Can you work these out from the model? Positions are in its coordinate system, mm. Give positions to 0.01 mm unless a question says otherwise; leave off trailing zeros. Loops run counter-clockwise (first coordinate to the right, second up) from the corner with the lowest first, then second, coordinate; pieces in that order, holes last. Notation, with made-up numbers: (-1, -2.5) - (54, -2.5) arc R18 cw to (54, 15.5) - close; hole circle Ø9 at (24, 44). An arc over 180 degrees is marked (long way). Write item = value, one per line.
from build123d import *

# Parameters (mm, degrees)
EXTRUSION3_DEPTH = 0.3
ESQUISSE2_W      = 12
ESQUISSE2_H      = 15
EXTRUSION4_DEPTH = 0.2


with BuildPart() as part:
    # Esquisse1 → Extrusion3 (new body)
    with BuildSketch(Plane.XY):
        with BuildLine():
            Line((-12.832841813, 25.021420219), (-12.832841813, 25.437540043))
            ThreePointArc((-12.832841813, 25.437540043), (-13.819409399, 26.424107629), (-14.805976985, 25.437540043))
            Line((-14.805976985, 25.437540043), (-14.805976985, 25.037540043))
            ThreePointArc((-14.805976985, 25.037540043), (-15.667751578, 24.60975507), (-16.333846188, 23.915512028))
            ThreePointArc((-16.333846188, 23.915512028), (-16.688617291, 23.169755053), (-16.810405862, 22.352942012))
            Line((-16.810405862, 22.352942012), (-16.810405862, 20.131551422))
            Line((-16.810405862, 20.131551422), (-17.410405862, 20.131551422))
            Line((-17.410405862, 20.131551422), (-17.410405862, 19.131551422))
            Line((-17.410405862, 19.131551422), (-14.810405862, 19.131551422))
            ThreePointArc((-14.810405862, 19.131551422), (-13.810405862, 18.131551422), (-12.810405862, 19.131551422))
            Line((-12.810405862, 19.131551422), (-10.210405862, 19.131551422))
            Line((-10.210405862, 19.131551422), (-10.210405862, 20.131551422))
            Line((-10.210405862, 20.131551422), (-10.810405862, 20.131551422))
            Line((-10.810405862, 20.131551422), (-10.810405862, 22.331551422))
            ThreePointArc((-10.810405862, 22.331551422), (-11.372418001, 24.014230931), (-12.832841813, 25.021420219))
        make_face()
        with BuildLine():
            Line((-11.310405862, 22.331551422), (-11.310405862, 19.631551422))
            Line((-11.310405862, 19.631551422), (-13.310405862, 19.631551422))
            Line((-13.310405862, 19.631551422), (-13.310405862, 19.131551422))
            ThreePointArc((-13.310405862, 19.131551422), (-13.810405862, 18.631551422), (-14.310405862, 19.131551422))
            Line((-14.310405862, 19.131551422), (-14.310405862, 19.631551422))
            Line((-14.310405862, 19.631551422), (-16.310405862, 19.631551422))
            Line((-16.310405862, 19.631551422), (-16.310405862, 22.352942012))
            ThreePointArc((-16.310405862, 22.352942012), (-16.21036525, 23.023895582), (-15.91894613, 23.636481668))
            ThreePointArc((-15.91894613, 23.636481668), (-15.220043493, 24.309156929), (-14.305976985, 24.633871146))
            Line((-14.305976985, 24.633871146), (-14.305976985, 25.437540043))
            ThreePointArc((-14.305976985, 25.437540043), (-13.819409399, 25.924107629), (-13.332841813, 25.437540043))
            Line((-13.332841813, 25.437540043), (-13.332841813, 24.614741777))
            ThreePointArc((-13.332841813, 24.614741777), (-11.888721032, 23.856609238), (-11.310405862, 22.331551422))
        make_face(mode=Mode.SUBTRACT)
    extrude(amount=EXTRUSION3_DEPTH)

    # Esquisse2 → Extrusion4 (add)
    with BuildSketch(Plane(origin=(0, 0, 0), x_dir=(-1, 0, 0), z_dir=(0, 0, -1))):
        with Locations((13.810405862, 22.167730135)):
            Rectangle(ESQUISSE2_W, ESQUISSE2_H)
    extrude(amount=EXTRUSION4_DEPTH)


solid = part.part
Q1. Imagine slicing it at A-A, the plane z = 0.15. Write out the boundary of the cut face in (x, y), then the cut area to 3 significant figures.
Output:
outline = (-17.41, 19.13) - (-14.81, 19.13) arc R1 ccw to (-12.81, 19.13) - (-10.21, 19.13) - (-10.21, 20.13) - (-10.81, 20.13) - (-10.81, 22.33) arc R2.8 ccw to (-12.83, 25.02) - (-12.83, 25.44) arc R0.99 ccw to (-14.81, 25.44) - (-14.81, 25.04) arc R2.8 ccw to (-16.81, 22.35) - (-16.81, 20.13) - (-17.41, 20.13) - close; hole (-16.31, 19.63) - (-14.31, 19.63) - (-14.31, 19.13) arc R0.5 ccw to (-13.31, 19.13) - (-13.31, 19.63) - (-11.31, 19.63) - (-11.31, 22.33) arc R2.3 ccw to (-13.33, 24.61) - (-13.33, 25.44) arc R0.49 ccw to (-14.31, 25.44) - (-14.31, 24.63) arc R2.3 ccw to (-16.31, 22.35) - close
area = 12.8 mm2
Q2. Imagine slicing it at D-D, the plane x = -13.75. Write out the boundary of the cut face in (y, z), then the cut area to 3 significant figures.
Output:
outline = (14.67, -0.2) - (29.67, -0.2) - (29.67, 0) - (26.42, 0) - (26.42, 0.3) - (25.92, 0.3) - (25.92, 0) - (18.64, 0) - (18.64, 0.3) - (18.13, 0.3) - (18.13, 0) - (14.67, 0) - close
area = 3.30 mm2
Q3. Imagine slicing it at B-B, the plane x = -17. Write out the boundary of the cut face in (y, z), then the cut area to 3 significant figures.
Output:
outline = (14.67, -0.2) - (29.67, -0.2) - (29.67, 0) - (20.13, 0) - (20.13, 0.3) - (19.13, 0.3) - (19.13, 0) - (14.67, 0) - close
area = 3.30 mm2
Q4. I need wall thicknesses on L1, parallel to X at y = 20, z = 0.1; L2, parallel to X at y = 21.75, z = 0.25; L3, parallel to Z at x = -16, y = 18.75. Which ranges of each line are inside material? Lowest first, please.
Output:
L1 = -17.41 to -16.31, -11.31 to -10.21
L2 = -16.81 to -16.31, -11.31 to -10.81
L3 = -0.2 to 0
Q5. We'd pull the mould along Y, two halves only. Please class faces 1 (the flat face through (-14, 22, 0)), 2 (the flat face through (-14, 22, -0.2)): released by +Y, released by -Y, zero draft, split by the parting line, or undercut.
Output:
face_1 = undercut
face_2 = zero draft
Q6. For pin 1 (1.5 mm diameter, centred on x = -13, y = 21.5, fed in from +Z); pin 2 (5 mm diameter, centred on x = -18, y = 19.5, fed in from +Z), each with a flat end and sliding along its axis, tell me the tip position at first contact or that it passes through.
Output:
pin_1 = 0
pin_2 = 0.3
Q7. Imagine slicing it at C-C, the plane y = 28.75. Write out the boundary of the cut face in (x, z).
Output:
outline = (-19.81, -0.2) - (-7.81, -0.2) - (-7.81, 0) - (-19.81, 0) - close
